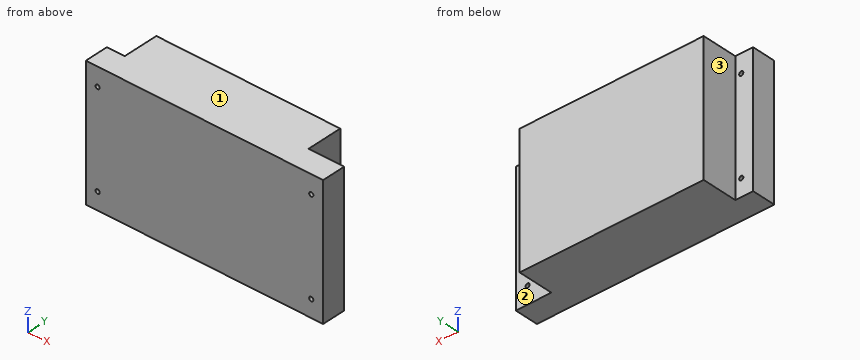
from build123d import *

# Parameters (mm, degrees)
SKETCH1_W           = 200
SKETCH1_H           = 110
BOSS_EXTRUDE1_DEPTH = 50
SKETCH2_W           = 30
SKETCH2_H           = 110
SKETCH2_W_2         = 15
CUT_EXTRUDE1_DEPTH  = 30
SKETCH3_R           = 1.75
CUT_EXTRUDE2_DEPTH  = 30


with BuildPart() as part:
    # Sketch1 → Boss-Extrude1 (new body)
    with BuildSketch(Plane(origin=(0, 0, 0), x_dir=(1, 0, 0), z_dir=(0, 1, 0))):
        with Locations((100, 55)):
            Rectangle(SKETCH1_W, SKETCH1_H)
    extrude(amount=BOSS_EXTRUDE1_DEPTH)

    # Sketch2 → Cut-Extrude1 (cut)
    with BuildSketch(Plane(origin=(0, 50, 0), x_dir=(1, 0, 0), z_dir=(0, 1, 0))):
        with Locations((185, 55)):
            Rectangle(SKETCH2_W, SKETCH2_H)
        with Locations((7.5, 55)):
            Rectangle(SKETCH2_W_2, SKETCH2_H)
    extrude(amount=-CUT_EXTRUDE1_DEPTH, mode=Mode.SUBTRACT)

    # Sketch3 → Cut-Extrude2 (cut)
    with BuildSketch(Plane(origin=(0, 20, 0), x_dir=(1, 0, 0), z_dir=(0, 1, 0))):
        with Locations((190, 95.5)):
            Circle(SKETCH3_R)
        with Locations((190, 15.5)):
            Circle(SKETCH3_R)
        with Locations((10, 95.5)):
            Circle(SKETCH3_R)
        with Locations((10, 15.5)):
            Circle(SKETCH3_R)
    extrude(amount=-CUT_EXTRUDE2_DEPTH, mode=Mode.SUBTRACT)


solid = part.part
Model file for the job. Use its own axes, mm. Face numbers are marked on the shaded views. A direction names the side the tool comes from. Give positions to 0.01 mm unless a question says otherwise; leave off trailing zeros. Order: outer loops, then holes, each group sorted by start corner. A loop starts at its lowest first (then second) coordinate and runs counter-clockwise, first axis right, second up. Notation, with made-up numbers: M 9.5,2.25 L 23.5,2.25 A22 ccw 23.5,35.25 Z; hole C 3,49.5 d3. An arc over 180 degrees is marked long. Put each result on its own line as item: value. Start each with the question number.
(1) Band-saw the part on A-A on z = -10.5. Give the cut face in (x, y).
(2) Drill centre lines: L1, parallel to Z at x = 190, y = 5; L2, parallel to X at y = 6.75, z = -95.5; L3, parallel to X at y = 42, z = -57. Where is each one in solid material? Low to high. Write a range as [from, to].
(3) Band-saw the part on B-B on y = 22. Give the cut face in (x, z), then the cut area to 4 significant figures.
(4) Pin check, flat tips, straight feed: pin 1 Ø1.5 at (y, z) = (43, -16.5) entering from +X; pin 2 Ø24 at (y, z) = (40, -77.5) entering from -X; pin 3 Ø4 at (x, z) = (190, -15.5) entering from +Y; pin 4 Ø1.5 at (x, y) = (76.5, 20.5) entering from +Z. Stop position of each tip, or through.
(5) Tool access for the marked faces 1, 2 and 3: list every direction of +Z, -Z, +X, -X, +Y, -Y with a clear straight run to the whole face (end or side of a thin tool).
Results below:
1. outline: M 0,0 L 200,0 L 200,20 L 170,20 L 170,50 L 15,50 L 15,20 L 0,20 Z
2. L1: z = [-110, -97.25], [-93.75, -17.25], [-13.75, 0]
2. L2: x = [0, 8.25], [11.75, 188.25], [191.75, 200]
2. L3: x = [15, 170]
3. outline: M 15,-110 L 170,-110 L 170,0 L 15,0 Z
3. area: 17,050 mm2
4. pin 1: stops at x = 170
4. pin 2: stops at x = 15
4. pin 3: stops at y = 20
4. pin 4: stops at z = 0
5. face 1: +Z, +X, -X, +Y, -Y
5. face 2: +Z, -Z, +X, +Y
5. face 3: +Z, -Z, -X, +Y
